The listing builds one solid part. Answer for the finished solid, in the listing's coordinates (mm). A direction names the side the tool comes from. Give positions to 0.01 mm unless a question says otherwise; leave off trailing zeros. Loops run counter-clockwise (first coordinate to the right, second up) from the corner with the lowest first, then second, coordinate; pieces in that order, holes last. Notation, with made-up numbers: (88.5, 75) - (120.5, 75) arc R31 ccw to (120.5, 105) - close; hole circle Ø1 at (-38.75, 11). An arc over 180 degrees is marked (long way). Answer in a Markdown table with one row per item. Add a question column.
```python
from build123d import *


with BuildPart() as f1:
    # F0 (on Front) → F1 (revolve)
    with BuildSketch(Plane.XZ):
        Polygon((-5.5380323902, 50.2795092762), (-30.604917556, 50.2795092762), (-46.0446093346, 54.9755878761), (-54.0652101429, 53.2870396276), (-56.2547557056, 63.687376678), (-67.3308223486, 61.3555721939), (-67.3308223486, 55.2345886827), (-62.3757392168, 55.2345886827), (-62.3757392168, 46.4903302491), (-37.6003272831, 39.7863946855), (-37.6003272831, 25.212623179), (-29.4390171766, 11.5132788196), (-29.4390171766, -6.8496726453), (-20.9862291813, -20.2575419098), (2.331804717, -12.0962299407), (11.3675408065, -29.8762302846), (31.1878658831, -23.4637726098), (18.0714763701, -13.5536063462), (22.1521314234, 11.2218027934), (36.7259047925, 29.8762302846), (36.7259047925, 45.3244261444), (9.9101634696, 49.4050830603), (-5.5380323902, 46.4903302491), align=None)
    revolve(axis=Axis((21.2777033448, 0, -26.6700014472), (-0.9514445247, 0, -0.3078202664)))


with BuildPart() as f4:
    # F3 (on Front) → F4 (revolve)
    with BuildSketch(Plane.XZ):
        Polygon((-49.0032210946, 49.8506426811), (-65.442211926, 49.8506426811), (-65.4422044754, 40.3364561498), (-60.2509491146, 40.3364561498), (-60.2509491146, 23.4703980386), (-33.4294438362, 23.4703980386), (-13.5296229273, 6.6043394618), (-13.5296229273, -6.8020136096), (0, -10.2617200464), (0, -87.2401446104), (15.8875081688, -87.2401446104), (15.8875081688, -115.782700479), (34.9221229553, -115.782700479), (34.9221229553, -85.077829659), (34.0569131076, -79.0233463049), (23.2417937368, -79.0233463049), (16.7527180165, -68.644233048), (4.6397843398, -68.644233048), (4.6397843398, -13.2889607921), (28.0004460365, -6.8020136096), (56.1197660863, 19.1457699984), (115.3866276145, 31.6872000694), (119.280077517, 49.8506426811), (127.0151686524, 49.8506426811), (127.0151686524, 58.6822458537), (115.3866276145, 60.6622211635), (111.9257882237, 40.3364561498), (95.2339635486, 40.3364561498), (91.3085111252, 49.6624633169), (80.1309212987, 44.9576527494), (82.0760503411, 40.3364561498), (40.9785918891, 23.0379365385), (32.3264971375, 9.6315825358), (0, 9.6315825358), (-20.88390477, 34.7144380212), (-49.0032210946, 34.7144380212), align=None)
    revolve(axis=Axis((25.4048155621, 0, -115.782700479), (-1, 0, 0)))


solid = f4.part
```
(1) Given pin 1 Ø4 at (x, z) = (86, -249) entering from +Y; pin 2 Ø6 at (x, z) = (-21.5, -215.5) entering from -Y; pin 3 Ø3 at (x, y) = (19, -46) entering from -Z, each flat-ended and moving along its own axis, determine where each tip first touches the part or whether it passes through.
(2) A cutting plane is placed at A-A on x = 49. Determine the outline of the cut face in (y, z), plus the area to 3 significant figures.
(3) Find the intervals of material crossed by line 1 along Z through (x, y) = (17, 13.5); line 2 along X through (y, z) = (-31.5, -274.5); line 3 along Z through (x, y) = (13, -43), in increasing order. Write a range as [from, to].
(4) A tool of negligible diameter and unlimited length cuts with its end or side. For faces 1 (the face through (34.922, 0, -115)), 2 (the face through (127.015, -154, -180)), 3 (the face through (94.988, -95.351, -240.136)), 4 (the face through (-62.81, 46.89, 33.13)), from which of +Z, -Z, +X, -X, +Y, -Y can it reach the whole face along a straight path? Write none if from no direction.
(5) The mould has two halves that part along Y. Classify faces 5 (the face through (22.836, 1.645, -153.155)), 6 (the face through (-65.442, 47.033, 33.568)), 7 (the face through (112.094, -153.37, -149.84)): pulls with the +Y half, pulls with the -Y half, needs draft (parallel to the pull), parting line crosses it, or undercut.
Evaluation:
| question | item | result |
|---|---|---|
| 1 | pin 1 | stops at y = 97.4 |
| 1 | pin 2 | stops at y = -115.3 |
| 1 | pin 3 | stops at z = -233.04 |
| 2 | outline | circle Ø284.39 at (0, -115.78); hole circle Ø256.72 at (0, -115.78) |
| 2 | area | 11,800 mm² |
| 3 | line 1 | z = [-240.47, -220.84], [-160.53, -71.03], [-10.72, 8.9] |
| 3 | line 2 | x = [-65.44, -49], [82.68, 92.84], [112.9, 118.46] |
| 3 | line 3 | z = [-233.6, -211.37], [-135.1, -96.47], [-20.19, 2.03] |
| 4 | face 1 | +X |
| 4 | face 2 | +Z, -Z, +X, +Y, -Y |
| 4 | face 3 | none |
| 4 | face 4 | -X |
| 5 | face 5 | undercut |
| 5 | face 6 | needs draft |
| 5 | face 7 | parting line crosses it |
